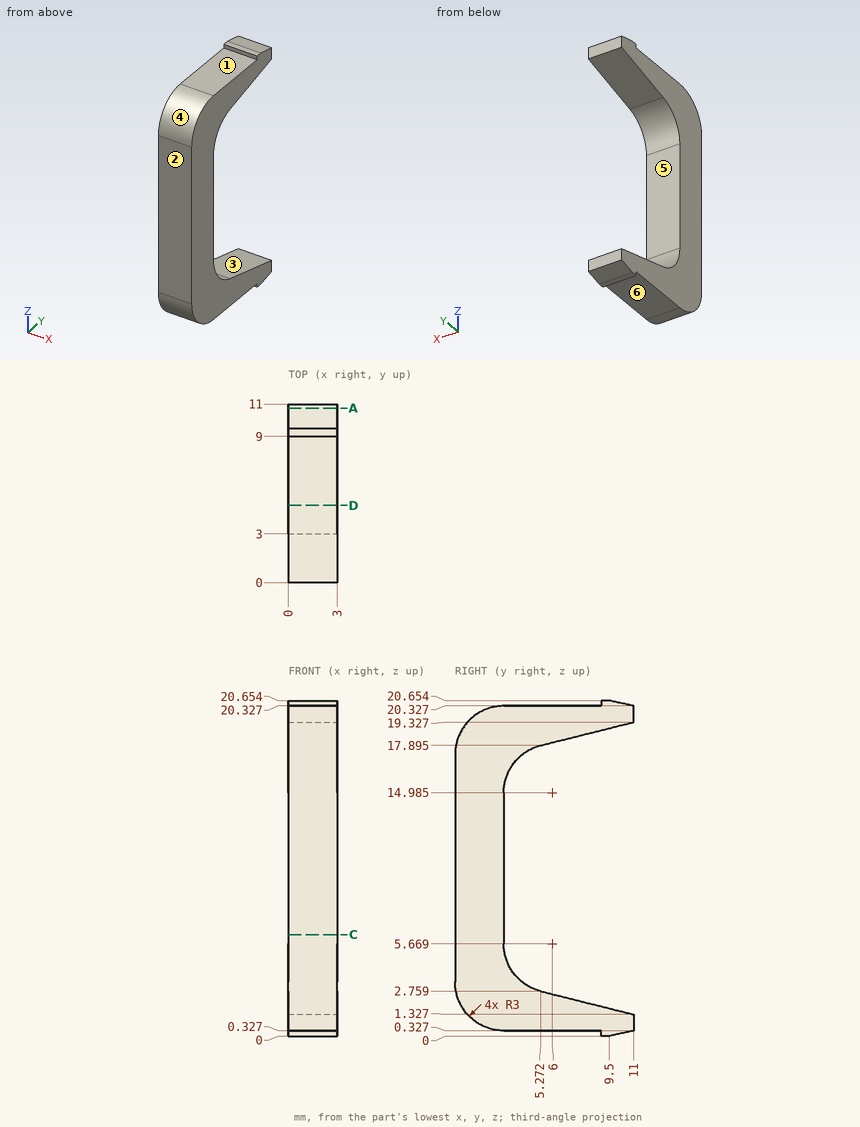
Part print with two shaded views. Sizes in mm from the minimum x, y, z corner. A direction names the side the tool comes from. Round coordinates to 2 decimals unless told otherwise and drop trailing zeros. Loops run counter-clockwise (first coordinate to the right, second up) from the corner with the lowest first, then second, coordinate; pieces in that order, holes last.
Item 1: Saw through at D-D (y = 4.75). List the corners of the cut face in (x, z), then the cut area to 3 significant figures.
Item 2: Saw through at A-A (y = 10.75). List the corners of the cut face in (x, z) (1 decimal).
Item 3: Which spindle directions (+Z, -Z, +X, -X, +Y, -Y) get a long thin tool onto all of the face, cutting with end or side? Do the marked faces 1, 2 and 3. Say none if no direction does.
Item 4: Saw through at C-C (z = 6.25). List the corners of the cut face in (x, y).
Item 5: Pin check, flat tip, straight feed: P1, Ø1.5, axis at x = 2, y = 4.5, coming from the +Z side. Stop position of the tip, or through.
Item 6: Drill centre lines: line 1 along Z through (x, y) = (2.4, 8); line 2 along Z through (x, y) = (0.55, 6); line 3 along Y through (x, z) = (2.3, 14.5). Where is each one in solid material? Low to high.
Item 7: Two-plate mould, pull along Z, no slides. Class the marked faces 4, 5 and 6: released by +Z, released by -Z, zero draft, split by the parting line, or undercut.
Worked answers:
1. outline: (0, 0.33) - (3, 0.33) - (3, 2.94) - (0, 2.94) - close; (0, 17.71) - (3, 17.71) - (3, 20.33) - (0, 20.33) - close
1. area: 15.7 mm2
2. outline: (0, 0.3) - (3, 0.3) - (3, 1.4) - (0, 1.4) - close; (0, 19.3) - (3, 19.3) - (3, 20.4) - (0, 20.4) - close
3. face 1: +Z, +X, -X, -Y
3. face 2: +Z, -Z, +X, -X, -Y
3. face 3: +X, -X, +Y
4. outline: (0, 0) - (3, 0) - (3, 3) - (0, 3) - close
5. P1: stops at z = 20.33
6. line 1: z = 0.33 to 2.08, 18.58 to 20.33
6. line 2: z = 0.33 to 2.58, 18.08 to 20.33
6. line 3: y = 0 to 3
7. face 4: released by +Z
7. face 5: undercut
7. face 6: released by -Z
